Geometry check sheet. Reference: the model listing, model coordinates, mm. A direction names the side the tool comes from. Round coordinates to 2 decimals unless told otherwise and drop trailing zeros. Order: outer loops, then holes, each group sorted by start corner. A loop starts at its lowest first (then second) coordinate and runs counter-clockwise, first axis right, second up.
(1) Cross-section at D-D on x = 6.5. Enter the section's corners in (y, z).
(2) Set-up check for faces 5 (the face through (2.15, 21, 4)), 6 (the face through (2.706, 39.322, 4.087)), 7 (the face through (7.9, 30.8, 4.6)), 8 (the face through (33, 9, 6.6)): record each of +Z, -Z, +X, -X, +Y, -Y from which the full face is reachable in a straight line by a thin tool's end or side.
(3) Cross-section at B-B on x = 16. Enter the section's corners in (y, z), and give its area (3 significant figures).
(4) Gauge pin test, flat ends, axial feed: P1, Ø0.5, axis at x = 34.5, z = 3, coming from the +Y side; P2, Ø0.5, axis at x = 31, z = 3, coming from the -Y side; P3, Ø1.1, axis at y = 4.5, z = 5, coming from the +X side. Record the tip position at first contact, or that the pin passes through.
(5) Cross-section at A-A on y = 34.5. Enter the section's corners in (x, z).
(6) Thickness scan on L1, parallel to X at y = 36.5, z = 4.7; L2, parallel to Z at x = 34, y = 10.5; L3, parallel to X at y = 22, z = 4.35. Record the ranges inside material, lowest first.
(7) Draft check along Z on faces 1 (the face through (39.294, 2.678, 4.087)), 2 (the face through (40.94, 21.24, 6.09)), 3 (the face through (9, 9, 6.6)), 4 (the face through (34, 35, 3.5)). Enter one of: pulls with the +Z half, pulls with the -Z half, needs draft (parallel to the pull), parting line crosses it, or undercut.
from build123d import *

# Parameters (mm, degrees)
PAD033_DEPTH    = 3.9
POCKET042_DEPTH = 2.2


with BuildPart() as part:
    # AdditivePipe007: sweep along a path in Sketch119
    with BuildLine(Plane.XY.offset(7.15)) as additivepipe007_path:
        ThreePointArc((42, 38), (40.828427, 40.828427), (38, 42))
        Line((38, 42), (4, 42))
        ThreePointArc((4, 42), (1.171573, 40.828427), (0, 38))
        Line((0, 38), (0, 4))
        ThreePointArc((0, 4), (1.171573, 1.171573), (4, 0))
        Line((4, 0), (38, 0))
        ThreePointArc((38, 0), (40.828427, 1.171573), (42, 4))
        Line((42, 4), (42, 38))
    # Sketch118 (on Sketch) → AdditivePipe007 (sweep)
    with BuildSketch(Plane.XZ.offset(-16)):
        Polygon((0, 7.15), (2.15, 5), (2.15, 3.2), (2.45, 2.9), (3.4, 2.9), (3.4, 7.15), align=None)
    sweep(path=additivepipe007_path.line)

    # Sketch138 → Pad033 (new body)
    with BuildSketch(Plane.XY.offset(2.7)):
        with BuildLine():
            Line((2.7, 27.6), (8, 27.6))
            ThreePointArc((8, 27.6), (12.525483, 29.474517), (14.4, 34))
            Line((14.4, 39.3), (14.4, 34))
            Line((14.4, 39.3), (2.7, 39.3))
            Line((2.7, 39.3), (2.7, 27.6))
        make_face()
        with BuildLine():
            Line((27.6, 39.3), (39.3, 39.3))
            Line((39.3, 39.3), (39.3, 27.6))
            Line((39.3, 27.6), (34, 27.6))
            ThreePointArc((27.6, 34), (29.474517, 29.474517), (34, 27.6))
            Line((27.6, 39.3), (27.6, 34))
        make_face()
        with BuildLine():
            Line((27.6, 8), (27.6, 2.7))
            Line((27.6, 2.7), (39.3, 2.7))
            Line((39.3, 2.7), (39.3, 14.4))
            Line((39.3, 14.4), (34, 14.4))
            ThreePointArc((34, 14.4), (29.474517, 12.525483), (27.6, 8))
        make_face()
        with BuildLine():
            Line((14.4, 8), (14.4, 2.7))
            Line((14.4, 2.7), (2.7, 2.7))
            Line((2.7, 2.7), (2.7, 14.4))
            Line((2.7, 14.4), (8, 14.4))
            ThreePointArc((14.4, 8), (12.525483, 12.525483), (8, 14.4))
        make_face()
    extrude(amount=PAD033_DEPTH)

    # Sketch149 → Pocket042 (cut)
    with BuildSketch(Plane.XY.offset(3.5)):
        with BuildLine():
            ThreePointArc((4.8, 34), (8, 30.8), (11.2, 34))
            Line((11.2, 34), (11.2, 42))
            Line((4.8, 42), (11.2, 42))
            Line((4.8, 34), (4.8, 42))
        make_face()
        with BuildLine():
            ThreePointArc((30.8, 34), (34, 30.8), (37.2, 34))
            Line((37.2, 34), (37.2, 42))
            Line((30.8, 42), (37.2, 42))
            Line((30.8, 34), (30.8, 42))
        make_face()
        with BuildLine():
            ThreePointArc((37.2, 8), (34, 11.2), (30.8, 8))
            Line((30.8, 8), (30.8, 0))
            Line((37.2, 0), (30.8, 0))
            Line((37.2, 8), (37.2, 0))
        make_face()
        with BuildLine():
            ThreePointArc((11.2, 8), (8, 11.2), (4.8, 8))
            Line((4.8, 8), (4.8, 0))
            Line((11.2, 0), (4.8, 0))
            Line((11.2, 8), (11.2, 0))
        make_face()
    extrude(amount=POCKET042_DEPTH, mode=Mode.SUBTRACT)


solid = part.part
Found:
1. outline: (0, 7.15) - (1.45, 5.7) - (10.83, 5.7) - (10.83, 3.5) - (2.15, 3.5) - (2.15, 3.2) - (2.45, 2.9) - (2.7, 2.9) - (2.7, 2.7) - (14.4, 2.7) - (14.4, 6.6) - (3.4, 6.6) - (3.4, 7.15) - close; (27.6, 2.7) - (39.3, 2.7) - (39.3, 2.9) - (39.55, 2.9) - (39.85, 3.2) - (39.85, 3.5) - (31.17, 3.5) - (31.17, 5.7) - (40.55, 5.7) - (42, 7.15) - (38.6, 7.15) - (38.6, 6.6) - (27.6, 6.6) - close
2. face 5: -Z, -X, +Y, -Y
2. face 6: -Z, -X, +Y
2. face 7: +Y
2. face 8: +Z
3. outline: (0, 7.15) - (2.15, 5) - (2.15, 3.2) - (2.45, 2.9) - (3.4, 2.9) - (3.4, 7.15) - close; (38.6, 2.9) - (39.55, 2.9) - (39.85, 3.2) - (39.85, 5) - (42, 7.15) - (38.6, 7.15) - close
3. area: 15.2 mm2
4. P1: stops at y = 39.85
4. P2: stops at y = 2.15
4. P3: stops at x = 40.4
5. outline: (0, 7.15) - (2.15, 5) - (2.15, 3.2) - (2.45, 2.9) - (2.7, 2.9) - (2.7, 2.7) - (14.4, 2.7) - (14.4, 6.6) - (3.4, 6.6) - (3.4, 7.15) - close; (27.6, 2.7) - (39.3, 2.7) - (39.3, 2.9) - (39.55, 2.9) - (39.85, 3.2) - (39.85, 5) - (42, 7.15) - (38.6, 7.15) - (38.6, 6.6) - (27.6, 6.6) - close; hole (4.8, 3.5) - (11.2, 3.5) - (11.2, 5.7) - (4.8, 5.7) - close; hole (30.8, 3.5) - (37.2, 3.5) - (37.2, 5.7) - (30.8, 5.7) - close
6. L1: x = 2.15 to 4.8, 11.2 to 14.4, 27.6 to 30.8, 37.2 to 39.85
6. L2: z = 2.7 to 3.5, 5.7 to 6.6
6. L3: x = 2.15 to 3.4, 38.6 to 39.85
7. face 1: needs draft
7. face 2: pulls with the -Z half
7. face 3: pulls with the +Z half
7. face 4: undercut
